from build123d import *

# Parameters (mm, degrees)
F1_DEPTH = 5
F0_W     = 70
F0_H     = 115
F0_W_2   = 45
F0_H_2   = 65
F0_W_3   = 100
F2_DEPTH = 10
F0_W_4   = 35
F0_H_3   = 55
F3_DEPTH = 10
F4_DEPTH = 5
F0_W_5   = 7
F0_H_4   = 35
F5_DEPTH = 8
F0_W_6   = 31
F6_DEPTH = 5
F0_H_5   = 2.5
F7_DEPTH = 5


with BuildPart() as f1:
    # F0 (on Front) → F1 (new body)
    with BuildSketch(Plane.XZ):
        Polygon((100, 60), (-100, 60), (-100, -60), (-90, -60), (-90, 55), (-20, 55), (-20, -60), (-10, -60), (-10, 55), (90, 55), (90, -60), (100, -60), align=None)
    extrude(amount=F1_DEPTH)

    # F0 (on Front) → F2 (join)
    with BuildSketch(Plane.XZ):
        with Locations((-55, -2.5)):
            Rectangle(F0_W, F0_H)
        Polygon((-70.5, -55), (-77.5, -55), (-77.5, -20), (-70.5, -20), (-70.5, -17.5), (-39.5, -17.5), (-39.5, -20), (-32.5, -20), (-32.5, -55), (-39.5, -55), align=None, mode=Mode.SUBTRACT)
        with Locations((-55, 17.5)):
            Rectangle(F0_W_2, F0_H_2, mode=Mode.SUBTRACT)
        with Locations((40, -2.5)):
            Rectangle(F0_W_3, F0_H)
    extrude(amount=F2_DEPTH)

    # F0 (on Front) → F3 (join)
    with BuildSketch(Plane.XZ):
        with Locations((-55, 17.5)):
            Rectangle(F0_W_2, F0_H_2)
        with Locations((-55, 17.5)):
            Rectangle(F0_W_4, F0_H_3, mode=Mode.SUBTRACT)
    extrude(amount=F3_DEPTH)

    # F0 (on Front) → F4 (cut)
    with BuildSketch(Plane.XZ):
        with Locations((-55, 17.5)):
            Rectangle(F0_W_2, F0_H_2)
        with Locations((-55, 17.5)):
            Rectangle(F0_W_4, F0_H_3, mode=Mode.SUBTRACT)
    extrude(amount=F4_DEPTH, mode=Mode.SUBTRACT)

    # F0 (on Front) → F5 (join)
    with BuildSketch(Plane.XZ):
        with Locations((-74, -37.5)):
            Rectangle(F0_W_5, F0_H_4)
        with Locations((-36, -37.5)):
            Rectangle(F0_W_5, F0_H_4)
    extrude(amount=F5_DEPTH)

    # F0 (on Front) → F6 (join)
    with BuildSketch(Plane.XZ):
        with Locations((-55, -37.5)):
            Rectangle(F0_W_6, F0_H_4)
    extrude(amount=F6_DEPTH)

    # F0 (on Front) → F7 (join)
    with BuildSketch(Plane.XZ):
        with Locations((-55, -18.75)):
            Rectangle(F0_W_6, F0_H_5)
    extrude(amount=F7_DEPTH)


solid = f1.part
Source: CAD feature listing. Evaluate the final solid. Frame: model axes, mm. A direction names the side the tool comes from. Give positions to 0.01 mm unless a question says otherwise; leave off trailing zeros. Write each loop counter-clockwise with the first axis right and the second up, starting at its lowest first coordinate (ties: lowest second). Pieces come first, ordered by that corner, then holes. Notation, with made-up numbers: M -31.75,-15 L -1.75,-15 A25 ccw -1.75,4 Z; hole C 22.25,5 d4. An arc over 180 degrees is marked long. Return JSON: item names as keys, results as strings. Group by question number.
1) Draft query along X for faces 1 (the face through (-1, -5, -60)), 2 (the face through (90, -7, -3)), 3 (the face through (-36, -8, -37)). Return one class per face: released by +X, released by -X, zero draft, split by the parting line, or undercut.
2) Ray query, L1, parallel to X at y = -8.25, z = 16; L2, parallel to X at y = -9.25, z = -50; L3, parallel to Z at x = -34.5, y = -4. Return the intervals inside material, ascending.
3) Set-up query: faces 4 (the face through (-20, -7, -3)), 5 (the face through (-77.5, -2, 17)), 6 (the face through (-55, -5, -36)), 7 (the face through (-55, -7, 55)). Return all of +Z, -Z, +X, -X, +Y, -Y with unobstructed straight access to the full face (end or side cutting, diameter ignored); none if empty.
4) First-contact query: pin 1 Ø3 at (y, z) = (-5.5, 42.5) entering from +X; pin 2 Ø1.5 at (y, z) = (-6.5, 17.5) entering from -X; pin 3 Ø6 at (x, z) = (-66.5, -31.5) entering from -Y; pin 4 Ø2 at (y, z) = (-8.5, 28) entering from +X. Flat tips, straight axial feed; report the tip coordinate or a pass-through.
5) Cut plane A-A, the plane x = -54. Output: boundary loops of the cut face in (y, z), then the cut area to 4 significant figures.
6) Cut plane B-B, the plane z = -5. Output: boundary loops of the cut face in (x, y), then the cut area to 3 significant figures.
7) Cut plane D-D, the plane z = -45.5. Output: boundary loops of the cut face in (x, y), then the cut area to 3 significant figures.
8) Cut plane C-C, the plane y = -2.75. Output: boundary loops of the cut face in (x, z), then the cut area to 3 significant figures.
Data:
{
 "1": {"face 1": "zero draft", "face 2": "released by +X", "face 3": "undercut"},
 "2": {"L1": "x = -90 to -72.5, -37.5 to -20, -10 to 90", "L2": "x = -90 to -77.5, -32.5 to -20, -10 to 90", "L3": "z = -60 to -15, 50 to 60"},
 "3": {"face 4": "+Z, -Z, -Y", "face 5": "+Y", "face 6": "-Y", "face 7": "+Z, +X, -X, -Y"},
 "4": {"pin 1": "stops at x = 100", "pin 2": "stops at x = -90", "pin 3": "stops at y = -5", "pin 4": "stops at x = 90"},
 "5": {"outline": "M -10,-60 L 0,-60 L 0,-15 L -5,-15 L -5,-10 L -10,-10 L -10,-17.5 L -5,-17.5 L -5,-55 L -10,-55 Z; M -10,45 L -5,45 L -5,50 L 0,50 L 0,60 L -5,60 L -5,55 L -10,55 Z", "area": "387.5 mm²"},
 "6": {"outline": "M -100,-5 L -90,-5 L -90,-10 L -72.5,-10 L -72.5,-5 L -77.5,-5 L -77.5,0 L -100,0 Z; M -37.5,-10 L -20,-10 L -20,-5 L -10,-5 L -10,-10 L 90,-10 L 90,-5 L 100,-5 L 100,0 L -32.5,0 L -32.5,-5 L -37.5,-5 Z", "area": "1,450 mm²"},
 "7": {"outline": "M -100,-5 L -90,-5 L -90,-10 L -77.5,-10 L -77.5,-8 L -70.5,-8 L -70.5,-5 L -39.5,-5 L -39.5,-8 L -32.5,-8 L -32.5,-10 L -20,-10 L -20,-5 L -10,-5 L -10,-10 L 90,-10 L 90,-5 L 100,-5 L 100,0 L -100,0 Z", "area": "1,670 mm²"},
 "8": {"outline": "M -100,-60 L 100,-60 L 100,60 L -100,60 Z; hole M -77.5,-15 L -32.5,-15 L -32.5,50 L -77.5,50 Z", "area": "21,100 mm²"}
}
